Here's how the part is built. I have some questions about the finished solid (model axes, mm). A direction names the side the tool comes from. Give positions to 0.01 mm unless a question says otherwise; leave off trailing zeros. Loops run counter-clockwise (first coordinate to the right, second up) from the corner with the lowest first, then second, coordinate; pieces in that order, holes last. Notation, with made-up numbers: (87.25, -3.75) - (118.25, -3.75) arc R14 cw to (118.25, 18.25) - close; hole circle Ø11 at (3.5, -9). An arc over 180 degrees is marked (long way). Put each result on its own line as item: value. Start each with the question number.
from build123d import *

# Parameters (mm, degrees)
F0_W     = 42.3
F0_H     = 42.3
F1_DEPTH = 28
F2_R     = 11
F3_DEPTH = 2
F4_R     = 2.5
F5_DEPTH = 24
F7_D     = 3
F8_SIZE  = 5.08


with BuildPart() as f1:
    # F0 (on Top) → F1 (new body)
    with BuildSketch(Plane.XY):
        Rectangle(F0_W, F0_H)
    extrude(amount=F1_DEPTH)

    # F2 (on face) → F3 (join)
    with BuildSketch(Plane.XY.offset(28)):
        Circle(F2_R)
    extrude(amount=F3_DEPTH)

    # F4 (on face) → F5 (join)
    with BuildSketch(Plane.XY.offset(28)):
        Circle(F4_R)
    extrude(amount=F5_DEPTH)

    # F7 (through all)
    with Locations(Plane(origin=(0, 0, 0), x_dir=(1, 0, 0), z_dir=(0, 0, -1))):
        with Locations((-16, 16), (16, 16), (-16, -16), (16, -16)):
            Hole(F7_D / 2)

    # F8
    f8_edges = [f1.edges().sort_by_distance(p)[0] for p in [
        (-21.15, -21.15, 14),
        (21.15, -21.15, 14),
        (21.15, 21.15, 14),
        (-21.15, 21.15, 14),
    ]]
    chamfer(f8_edges, length=F8_SIZE)


solid = f1.part
1) Which directions (+Z, -Z, +X, -X, +Y, -Y) give clear straight access to the entire face, cutting with the end or side of a thin tool? Please do faces 1 (the cylindrical face through (-0.54, -2.44, 40.85)), 2 (the flat face through (-21.15, 0, 14)).
2) I need wall thicknesses on line 1 (Y direction, x = 16, z = 8.5); line 2 (Y direction, x = 15.5, z = 8). Which ranges of each line are inside material? Lowest first, please.
3) Suppose I cut it at D-D on z = 32.5. Please give me the cut outline in (x, y), plus the area to 3 significant figures.
4) Suppose I cut it at B-B on y = 0. Please give me the cut outline in (x, z).
5) Thinking about a two-plate mould opening in X: for faces 3 (the flat face through (0, 0, 52)), 4 (the flat face through (-18.57, -18.65, 13.8)), 5 (the cylindrical face through (-14.5, -16.07, 14.2)), 6 (the cylindrical face through (-2.38, -10.74, 28.99)), which applies, pulls with the +X half, pulls with the -X half, needs draft (parallel to the pull), parting line crosses it, or undercut?
6) I'm going to push flat-ended pins straight in: P1, Ø8, axis at y = 4, z = 46.5, coming from the -X side; P2, Ø1.5, axis at x = -3.5, y = 10.5, coming from the +Z side; P3, Ø10, axis at y = 5, z = 33.5, coming from the -X side. Where does each tip first touch, or does it pass through?
7) Suppose I cut it at A-A on z = 5. Please give me the cut outline in (x, y).
Ans:
1. face 1: +Z
1. face 2: +Z, -Z, -X, +Y, -Y
2. line 1: y = -21.15 to -17.5, -14.5 to 14.5, 17.5 to 21.15
2. line 2: y = -21.15 to -17.41, -14.59 to 14.59, 17.41 to 21.15
3. outline: circle Ø5 at (0, 0)
3. area: 19.6 mm²
4. outline: (-21.15, 0) - (21.15, 0) - (21.15, 28) - (11, 28) - (11, 30) - (2.5, 30) - (2.5, 52) - (-2.5, 52) - (-2.5, 30) - (-11, 30) - (-11, 28) - (-21.15, 28) - close
5. face 3: needs draft
5. face 4: pulls with the -X half
5. face 5: undercut
5. face 6: parting line crosses it
6. P1: stops at x = -2.5
6. P2: stops at z = 30
6. P3: stops at x = -10.91
7. outline: (-21.15, -16.07) - (-16.07, -21.15) - (16.07, -21.15) - (21.15, -16.07) - (21.15, 16.07) - (16.07, 21.15) - (-16.07, 21.15) - (-21.15, 16.07) - close; hole circle Ø3 at (-16, -16); hole circle Ø3 at (-16, 16); hole circle Ø3 at (16, -16); hole circle Ø3 at (16, 16)
